from build123d import *

# Parameters (mm, degrees)
BOSS_EXTRUDE1_DEPTH         = 2.54
CUT_EXTRUDE1_DEPTH          = 3.54
SKETCH7_W                   = 177.8
SKETCH7_H                   = 66.675
CUT_EXTRUDE2_DEPTH          = 3.54
F_27_0_144_DIAMETER_HOLE1_D = 3.6576


with BuildPart() as part:
    # Sketch1 → Boss-Extrude1 (new body)
    with BuildSketch(Plane(origin=(0, 0, 0), x_dir=(0, 1, 0), z_dir=(0, 0, 1))):
        with BuildLine():
            Line((-107.9246, -99.568), (107.9246, -99.568))
            ThreePointArc((107.9246, -99.568), (119.976103714, -94.576103714), (124.968, -82.5246))
            Line((124.968, -82.5246), (124.968, 82.5246))
            ThreePointArc((124.968, 82.5246), (119.976103714, 94.576103714), (107.9246, 99.568))
            Line((107.9246, 99.568), (-107.9246, 99.568))
            ThreePointArc((-107.9246, 99.568), (-119.976103714, 94.576103714), (-124.968, 82.5246))
            Line((-124.968, 82.5246), (-124.968, -82.5246))
            ThreePointArc((-124.968, -82.5246), (-119.976103714, -94.576103714), (-107.9246, -99.568))
        make_face()
    extrude(amount=BOSS_EXTRUDE1_DEPTH)

    # Sketch6 → Cut-Extrude1 (cut, through all)
    with BuildSketch(Plane.XY.offset(2.54)):
        with BuildLine():
            Line((49.8475, 4.691829089), (49.8475, -0.9525))
            Line((49.8475, -0.9525), (-57.4675, -0.9525))
            Line((-57.4675, -0.9525), (-57.4675, -11.7475))
            Line((-57.4675, -11.7475), (47.961208895, -11.7475))
            ThreePointArc((47.961208895, -11.7475), (53.34, -13.97), (58.718791105, -11.7475))
            Line((58.718791105, -11.7475), (63.1825, -11.7475))
            Line((63.1825, -11.7475), (63.1825, -0.9525))
            Line((63.1825, -0.9525), (56.8325, -0.9525))
            Line((56.8325, -0.9525), (56.8325, 4.691829089))
            ThreePointArc((56.8325, 4.691829089), (68.58, 19.52625), (56.8325, 34.360670911))
            Line((56.8325, 34.360670911), (56.8325, 40.64))
            Line((56.8325, 40.64), (69.85, 40.64))
            Line((69.85, 40.64), (69.85, 104.14))
            Line((69.85, 104.14), (36.83, 104.14))
            Line((36.83, 104.14), (36.83, 40.64))
            Line((36.83, 40.64), (49.8475, 40.64))
            Line((49.8475, 40.64), (49.8475, 34.360670911))
            ThreePointArc((49.8475, 34.360670911), (38.1, 19.52625), (49.8475, 4.691829089))
        make_face()
        with BuildLine():
            ThreePointArc((-25.732344403, 44.796363636), (-38.1, 97.79), (-50.467655597, 44.796363636))
            ThreePointArc((-50.467655597, 44.796363636), (-38.1, 29.21), (-25.732344403, 44.796363636))
        make_face()
    extrude(amount=-CUT_EXTRUDE1_DEPTH, mode=Mode.SUBTRACT)

    # Sketch7 → Cut-Extrude2 (cut, through all)
    with BuildSketch(Plane.XY.offset(2.54)):
        with Locations((0, -50.3555)):
            Rectangle(SKETCH7_W, SKETCH7_H)
    extrude(amount=-CUT_EXTRUDE2_DEPTH, mode=Mode.SUBTRACT)

    # #27 (0.144) Diameter Hole1 (through all)
    with Locations(Plane.XY.offset(2.54)):
        with Locations((93.8276, 0), (-93.8276, 0), (47.244, -119.2276), (-47.244, -119.2276), (93.8276, -83.6676), (-93.8276, -83.6676), (-93.8276, 83.6676), (93.8276, 83.6676), (-47.244, 119.2276), (47.244, 119.2276)):
            Hole(F_27_0_144_DIAMETER_HOLE1_D / 2)


solid = part.part
Geometry check sheet. Reference: the model listing, model coordinates, mm. A direction names the side the tool comes from. Round coordinates to 2 decimals unless told otherwise and drop trailing zeros. Order: outer loops, then holes, each group sorted by start corner. A loop starts at its lowest first (then second) coordinate and runs counter-clockwise, first axis right, second up. Notation, with made-up numbers: M 13.5,59 L 29.5,59 A29 cw 29.5,87 Z; hole C 16,-11.5 d3. An arc over 180 degrees is marked long. Write each question's results on one line, items separated by ' | '. Start each with the question number.
1. Set-up check for faces 5 (the face through (38.103, 19.812, 1.288)), 6 (the face through (-1, 26, 2.54)): record each of +Z, -Z, +X, -X, +Y, -Y from which the full face is reachable in a straight line by a thin tool's end or side.
2. Cross-section at A-A on y = -73.5. Record the boundary of the cut face in (x, z).
3. Material ranges on L1, parallel to Y at x = 10, z = 1.8; L2, parallel to Y at x = -38.1, z = 1.4; L3, parallel to X at y = -76, z = 2.2, recorded low to high. Write a range as from..to.
4. Draft check along X on faces 1 (the face through (-37.05, 97.77, 1.29)), 2 (the face through (-94.44, 120.11, 1.25)), 3 (the face through (94.44, -120.11, 1.25)), 4 (the face through (-1, 26, 0)). Enter one of: pulls with the +X half, pulls with the -X half, needs draft (parallel to the pull), parting line crosses it, or undercut.
5. Cross-section at B-B on x = -38.1. Record the boundary of the cut face in (y, z), plus the area to 3 significant figures.
6. Cross-section at D-D on z = 0.4. Give the number of separate pieces and of enclosed holes in the cut face, plus the area to 3 significant figures.
7. Cross-section at C-C on y = 69.85. Record the boundary of the cut face in (x, z).
Resolved:
1) face 5: +Z, -Z | face 6: +Z, +X, -X, +Y, -Y
2) outline: M -99.57,0 L -88.9,0 L -88.9,2.54 L -99.57,2.54 Z; M 88.9,0 L 99.57,0 L 99.57,2.54 L 88.9,2.54 Z
3) L1: -124.97..-83.69, -17.02..-11.75, -0.95..124.97 | L2: -124.97..-83.69, -17.02..-11.75, -0.95..29.21, 97.79..124.97 | L3: -99.57..-88.9, 88.9..99.57
4) face 1: undercut | face 2: pulls with the -X half | face 3: pulls with the +X half | face 4: needs draft
5) outline: M -124.97,0 L -83.69,0 L -83.69,2.54 L -124.97,2.54 Z; M -17.02,0 L -11.75,0 L -11.75,2.54 L -17.02,2.54 Z; M -0.95,0 L 29.21,0 L 29.21,2.54 L -0.95,2.54 Z; M 97.79,0 L 124.97,0 L 124.97,2.54 L 97.79,2.54 Z | area: 264 mm2
6) separate pieces: 1 | enclosed holes: 13 | area: 30,600 mm2
7) outline: M -99.57,0 L -66.04,0 L -66.04,2.54 L -99.57,2.54 Z; M -10.16,0 L 36.83,0 L 36.83,2.54 L -10.16,2.54 Z; M 69.85,0 L 99.57,0 L 99.57,2.54 L 69.85,2.54 Z
